from build123d import *


with BuildPart() as part:
    # Esquisse1 → Révolution1 (revolve)
    with BuildSketch(Plane.XY, mode=Mode.PRIVATE) as r_volution1_sk:
        with BuildLine():
            Line((17.923212734, 6.5), (19.131924887, 6.5))
            Line((19.131924887, 6.5), (19.131924887, 4.5))
            ThreePointArc((19.131924887, 4.5), (18.985478277, 4.146446609), (18.631924887, 4))
            Line((18.631924887, 4), (12.631924887, 4))
            ThreePointArc((12.631924887, 4), (12.278371496, 4.146446609), (12.131924887, 4.5))
            Line((12.131924887, 4.5), (12.131924887, 6.5))
            Line((12.131924887, 6.5), (13.340637039, 6.5))
            ThreePointArc((13.340637039, 6.5), (15.631924887, 5), (17.923212734, 6.5))
        make_face()
    revolve(r_volution1_sk.sketch.rotate(Axis((0, 0, 0), (1, 0, 0)), 90), axis=Axis((0, 0, 0), (1, 0, 0)))


solid = part.part
Verification items for the finished model (mm, model axes). Coordinates: 2 decimals unless noted, no trailing zeros. Order: outer loops, then holes, each group sorted by start corner. A loop starts at its lowest first (then second) coordinate and runs counter-clockwise, first axis right, second up. Notation, with made-up numbers: M 25,-9.75 L 73,-9.75 A31 cw 73,18.25 Z; hole C 45.25,75.25 d7. An arc over 180 degrees is marked long. One line per item, written item: value. Start each with the question number.
Item 1: Mould release check, pull along Z, two halves, no side actions. Record for faces 1 (the cylindrical face through (18.536, 3.955, -5.158)), 2 (the cylindrical face through (15.59, 3.905, -0.867)), 3 (the flat face through (12.132, -1.54, 4.42)): pulls with the +Z half, pulls with the -Z half, needs draft (parallel to the pull), parting line crosses it, or undercut.
Item 2: Sectioned sample at A-A on y = 0. Record the cut outline in (x, z).
Item 3: Sectioned sample at C-C on x = 13. Record the cut outline in (y, z), then the cut area to 3 significant figures.
Item 4: Depth check by flat-ended pin: P1, Ø2, axis at x = 13.5, z = -1.5, coming from the +Y side; P2, Ø1, axis at x = 15, z = 2.5, coming from the -Y side; P3, Ø1, axis at y = -1.5, z = -3.5, coming from the -X side. Enter the tip coordinate at first touch or a pass-through.
Item 5: Sectioned sample at D-D on x = 13.75. Record the cut outline in (y, z).
Item 6: Thickness scan on probe 1 along X at (y, z) = (1, 5.75); probe 2 along Z at (x, y) = (15.75, 2.5); probe 3 along Y at (x, z) = (17.45, 0). Record the ranges inside material, lowest first.
Calculated:
1. face 1: parting line crosses it
1. face 2: undercut
1. face 3: needs draft
2. outline: M 12.13,-6.5 L 13.34,-6.5 A2.5 cw 17.92,-6.5 L 19.13,-6.5 L 19.13,-4.5 A0.5 ccw 18.63,-4 L 12.63,-4 A0.5 ccw 12.13,-4.5 Z; M 12.13,4.5 A0.5 ccw 12.63,4 L 18.63,4 A0.5 ccw 19.13,4.5 L 19.13,6.5 L 17.92,6.5 A2.5 cw 13.34,6.5 L 12.13,6.5 Z
3. outline: C 0,0 d13; hole C 0,0 d8
3. area: 82.5 mm^2
4. P1: y = 6.48
4. P2: y = -4.74
4. P3: x = 12.17
5. outline: C 0,0 d11.71; hole C 0,0 d8
6. probe 1: 12.13 to 13.77, 17.5 to 19.13
6. probe 2: -4.33 to -3.12, 3.12 to 4.33
6. probe 3: -5.78 to -4, 4 to 5.78
